from build123d import *

# Parameters (mm, degrees)
F0_R     = 2.3114
F0_W     = 3.175
F0_H     = 160
F1_DEPTH = 3.175


with BuildPart() as f1:
    # F0 (on Top) → F1 (new body)
    with BuildSketch(Plane.XY):
        Polygon((-150, -150), (150, -150), (150, 150), (50, 150), (-50, 150), (-150, 150), align=None)
        with Locations((-50, -137.5)):
            Circle(F0_R, mode=Mode.SUBTRACT)
        with Locations((-137.5, -50)):
            Circle(F0_R, mode=Mode.SUBTRACT)
        with Locations((-101.5875, 0)):
            Rectangle(F0_W, F0_H, mode=Mode.SUBTRACT)
        with Locations((-30, -26.575)):
            Circle(F0_R, mode=Mode.SUBTRACT)
        with Locations((50, -137.5)):
            Circle(F0_R, mode=Mode.SUBTRACT)
        with Locations((30, -26.575)):
            Circle(F0_R, mode=Mode.SUBTRACT)
        with Locations((137.5, -50)):
            Circle(F0_R, mode=Mode.SUBTRACT)
        with Locations((101.5875, 0)):
            Rectangle(F0_W, F0_H, mode=Mode.SUBTRACT)
        with Locations((-137.5, 50)):
            Circle(F0_R, mode=Mode.SUBTRACT)
        with Locations((-60, 18.970938)):
            Circle(F0_R, mode=Mode.SUBTRACT)
        with BuildLine():
            ThreePointArc((-47.6886, 137.5), (-51.634407, 135.865593), (-50, 139.8114))
            ThreePointArc((-50, 139.8114), (-48.365593, 139.134407), (-47.6886, 137.5))
        make_face(mode=Mode.SUBTRACT)
        with Locations((60, 18.970938)):
            Circle(F0_R, mode=Mode.SUBTRACT)
        with Locations((137.5, 50)):
            Circle(F0_R, mode=Mode.SUBTRACT)
        with BuildLine():
            ThreePointArc((52.3114, 137.5), (50, 135.1886), (47.6886, 137.5))
            ThreePointArc((47.6886, 137.5), (48.365593, 139.134407), (50, 139.8114))
            ThreePointArc((50, 139.8114), (51.634407, 139.134407), (52.3114, 137.5))
        make_face(mode=Mode.SUBTRACT)
    extrude(amount=F1_DEPTH)


solid = f1.part
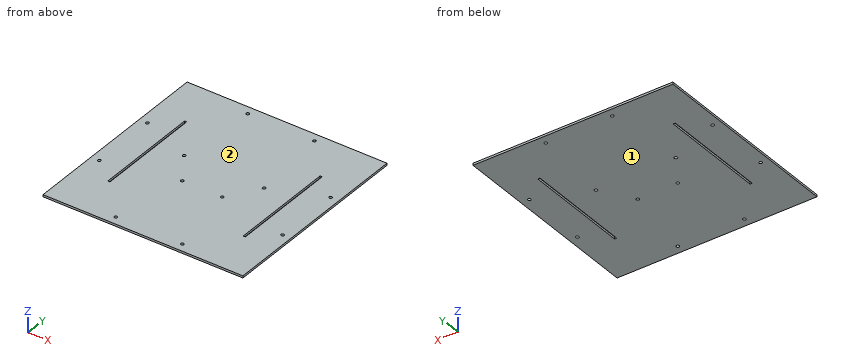
Geometry check sheet. Reference: the model listing, model coordinates, mm. Face numbers are marked on the shaded views. Give positions to 0.01 mm unless a question says otherwise; leave off trailing zeros. Order: outer loops, then holes, each group sorted by start corner. A loop starts at its lowest first (then second) coordinate and runs counter-clockwise, first axis right, second up.
1) Material ranges on probe 1 along X at (y, z) = (-8, 2.95) (3 decimals); probe 2 along Y at (x, z) = (137.5, 1.5); probe 3 along X at (y, z) = (49.5, 2.25) (3 decimals), recorded low to high.
Results are:
probe 1: x = -150 to -103.175, -100 to 100, 103.175 to 150
probe 2: y = -150 to -52.31, -47.69 to 47.69, 52.31 to 150
probe 3: x = -150 to -139.757, -135.243 to -103.175, -100 to 100, 103.175 to 135.243, 139.757 to 150
2) Gauge pin test, flat end, axial feed: pin 1 (6 mm diameter, centred on x = 60, y = 18.97, fed in from -Z). Record the tip position at first contact, or that the pin passes through.
Results are:
pin 1: stops at z = 0
3) Cross-section at A-A (y = 33.5). Record the boundary of the cut face in (x, z) (3 decimals), then the cut area to 3 significant figures.
Results are:
outline: (-150, 0) - (-103.175, 0) - (-103.175, 3.175) - (-150, 3.175) - close; (-100, 0) - (100, 0) - (100, 3.175) - (-100, 3.175) - close; (103.175, 0) - (150, 0) - (150, 3.175) - (103.175, 3.175) - close
area: 932 mm2
4) Draft check along Z on the marked faces 1 and 2. Enter one of: released by +Z, released by -Z, zero draft, split by the parting line, or undercut.
Results are:
face 1: released by -Z
face 2: released by +Z
